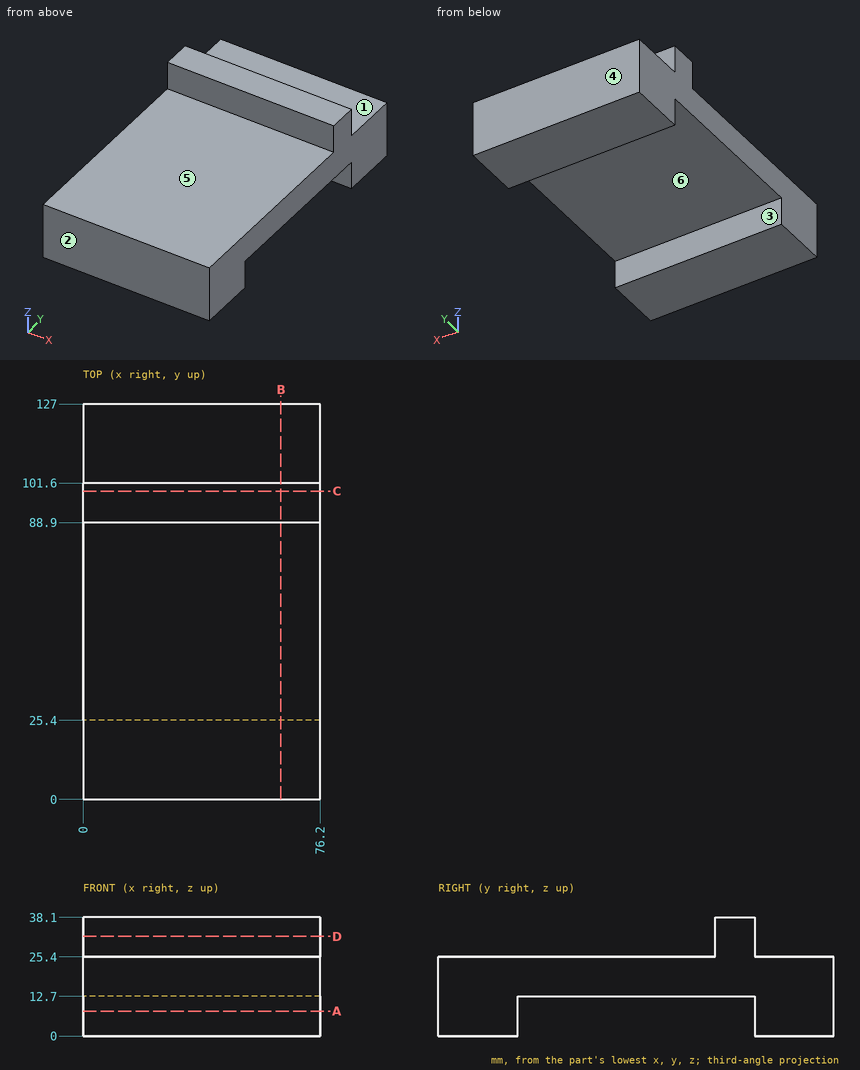
Input: dimensioned drawing with shaded views. Units: mm. Origin: part minimum x, y, z. A direction names the side the tool comes from. Coordinates: 2 decimals unless noted, no trailing zeros. Loops run counter-clockwise (first coordinate to the right, second up) from the corner with the lowest first, then second, coordinate; pieces in that order, holes last.
Q1. Section C-C, the plane y = 99. Return the cut outline in (x, z), and give its area (3 significant figures).
Results are:
outline: (0, 12.7) - (76.2, 12.7) - (76.2, 38.1) - (0, 38.1) - close
area: 1,940 mm2
Q2. Section B-B, the plane x = 63.5. Return the cut outline in (y, z).
Results are:
outline: (0, 0) - (25.4, 0) - (25.4, 12.7) - (101.6, 12.7) - (101.6, 0) - (127, 0) - (127, 25.4) - (101.6, 25.4) - (101.6, 38.1) - (88.9, 38.1) - (88.9, 25.4) - (0, 25.4) - close
Q3. Set-up query: the marked faces 4, 5 and 6. Return all of +Z, -Z, +X, -X, +Y, -Y with unobstructed straight access to the full face (end or side cutting, diameter ignored); none if empty.
Results are:
face 4: +Z, -Z, +X, -X, +Y
face 5: +Z, +X, -X, -Y
face 6: -Z, +X, -X
Q4. Section D-D, the plane z = 32. Return the cut outline in (x, y).
Results are:
outline: (0, 88.9) - (76.2, 88.9) - (76.2, 101.6) - (0, 101.6) - close
Q5. Section A-A, the plane z = 8. Return the cut outline in (x, y), and give its area (3 significant figures).
Results are:
outline: (0, 0) - (76.2, 0) - (76.2, 25.4) - (0, 25.4) - close; (0, 101.6) - (76.2, 101.6) - (76.2, 127) - (0, 127) - close
area: 3,870 mm2
Q6. Line query: line 1 along Y through (x, z) = (61, 8); line 2 along Z through (x, y) = (59, 121); line 3 along Z through (x, y) = (10, 30). Output: solid intervals per line, ascending.
Results are:
line 1: y = 0 to 25.4, 101.6 to 127
line 2: z = 0 to 25.4
line 3: z = 12.7 to 25.4
Q7. Contact query for flat-ended pins moving along their axis: pin 1 (10 mm diameter, centred on x = 48.5, y = 78, fed in from +Z); pin 2 (6.5 mm diameter, centred on x = 35.5, z = 34.5, fed in from +Y); pin 3 (10 mm diameter, centred on x = 58, y = 92, fed in from -Z). Output: stop coordinate, or through.
Results are:
pin 1: stops at z = 25.4
pin 2: stops at y = 101.6
pin 3: stops at z = 12.7
Q8. Mould query, pull axis Y, two halves, no side actions, for the marked faces 1, 2 and 3. Classes: +Y half, -Y half, draft (parallel to the pull), parting line (faces both ways), or undercut.
Results are:
face 1: draft
face 2: -Y half
face 3: undercut
